```python
from build123d import *

# Parameters (mm, degrees)
SKETCH1_R           = 11
SKETCH1_R_2         = 1.5
SKETCH1_W           = 5
SKETCH1_H           = 6
BOSS_EXTRUDE1_DEPTH = 5


with BuildPart() as part:
    # Sketch1 → Boss-Extrude1 (new body)
    with BuildSketch(Plane(origin=(0, 0, 0), x_dir=(1, 0, 0), z_dir=(0, 1, 0))):
        with BuildLine():
            Line((48.7, 25.000004028), (38.700001305, 25.000004028))
            ThreePointArc((38.700001305, 25.000004028), (35.164467017, 23.535538857), (33.7, 20.000005334))
            Line((33.7, 20.000005334), (33.7, -25))
            ThreePointArc((33.7, -25), (35.164465799, -28.535533784), (38.699999411, -30))
            Line((38.699999411, -30), (54.2, -30))
            Line((54.2, -30), (54.2, -55))
            Line((54.2, -55), (41.099999997, -55))
            Line((41.099999997, -55), (41.099999997, -63))
            Line((41.099999997, -63), (-23.900000003, -63))
            Line((-23.900000003, -63), (-23.900000003, -55))
            Line((-23.900000003, -55), (-37.00036842, -55))
            ThreePointArc((-37.00036842, -55), (-42.656802211, -52.657122122), (-45.000000024, -47.000820858))
            Line((-45.000000024, -47.000820858), (-45.000000024, 15.001139744))
            ThreePointArc((-45.000000024, 15.001139744), (-36.213537283, 36.213537259), (-15.001139768, 45))
            Line((-15.001139768, 45), (48.7, 45))
            ThreePointArc((48.7, 45), (58.699997986, 35.000002014), (48.7, 25.000004028))
        make_face()
        Circle(SKETCH1_R, mode=Mode.SUBTRACT)
        with Locations((9.89288341, 9.906102051)):
            Circle(SKETCH1_R_2, mode=Mode.SUBTRACT)
        with Locations((9.89288341, -9.906102051)):
            Circle(SKETCH1_R_2, mode=Mode.SUBTRACT)
        with Locations((-9.89288341, -9.906102051)):
            Circle(SKETCH1_R_2, mode=Mode.SUBTRACT)
        with Locations((-9.89288341, 9.906102051)):
            Circle(SKETCH1_R_2, mode=Mode.SUBTRACT)
        with Locations((-9.400000003, -59)):
            Circle(SKETCH1_R_2, mode=Mode.SUBTRACT)
        with Locations((26.599999997, -59)):
            Circle(SKETCH1_R_2, mode=Mode.SUBTRACT)
        with Locations((48.7, 35.000002014)):
            Circle(SKETCH1_R_2, mode=Mode.SUBTRACT)
        with Locations((-30.000000024, -40)):
            Circle(SKETCH1_R_2, mode=Mode.SUBTRACT)
        with Locations((36.599999976, -40)):
            Circle(SKETCH1_R_2, mode=Mode.SUBTRACT)
        with Locations((-39.500000024, -31)):
            Rectangle(SKETCH1_W, SKETCH1_H, mode=Mode.SUBTRACT)
        with Locations((-39.500000024, -47)):
            Rectangle(SKETCH1_W, SKETCH1_H, mode=Mode.SUBTRACT)
        with Locations((48.7, -36)):
            Rectangle(SKETCH1_W, SKETCH1_H, mode=Mode.SUBTRACT)
        with Locations((48.7, -49)):
            Rectangle(SKETCH1_W, SKETCH1_H, mode=Mode.SUBTRACT)
    extrude(amount=BOSS_EXTRUDE1_DEPTH)


solid = part.part
```
Geometry check sheet. Reference: the model listing, model coordinates, mm. A direction names the side the tool comes from. Coordinates: 2 decimals unless noted, no trailing zeros. Write each loop counter-clockwise with the first axis right and the second up, starting at its lowest first coordinate (ties: lowest second). Pieces come first, ordered by that corner, then holes. Notation, with made-up numbers: M -4,17.25 L 13,17.25 A9 ccw 13,32.25 Z; hole C 86,65.5 d6. An arc over 180 degrees is marked long. Answer as a JSON object with one key per item and string values.
1. Section check D-D, the plane z = -17. Enter the section's corners in (x, y), plus the area to 3 significant figures.
Answers below:
{"outline": "M -44.93,0 L 33.7,0 L 33.7,5 L -44.93,5 Z", "area": "393 mm²"}
2. Section check B-B, the plane x = 36.6. Enter the section's corners in (y, z), plus the area to 3 significant figures.
Answers below:
{"outline": "M 0,-45 L 5,-45 L 5,-24.54 L 0,-24.54 Z; M 0,29.54 L 5,29.54 L 5,38.5 L 0,38.5 Z; M 0,41.5 L 5,41.5 L 5,63 L 0,63 Z", "area": "255 mm²"}
3. Tool access check on faces 4 (the flat face through (44, 2, -25)), 5 (the flat face through (-30, 2, 55)), 6 (the flat face through (48, 2, 55)), 7 (the flat face through (-40, 2, 50)). Record the directions out of +Z, -Z, +X, -X, +Y, -Y that give a thin tool (end or side, any length) a straight path to the whole face; none if there is none.
Answers below:
{"face 4": "+X, +Y, -Y", "face 5": "+Z, -X, +Y, -Y", "face 6": "+Z, +X, +Y, -Y", "face 7": "+Y, -Y"}
4. Go/stop test with flat-tipped pins: pin 1 Ø2.5 at (y, z) = (2, 2) entering from +X; pin 2 Ø2.5 at (x, y) = (49, 3) entering from +Z; pin 3 Ø1 at (y, z) = (4, -22) entering from +X; pin 4 Ø20 at (x, z) = (0, 0) entering from +Y. Record where each tip stops, or that it passes through.
Answers below:
{"pin 1": "stops at x = 33.7", "pin 2": "stops at z = 55", "pin 3": "stops at x = 34.37", "pin 4": "passes through"}
5. Scan lines: L1, parallel to X at y = 3.4, z = 59; L2, parallel to Z at x = 48.7, y = 3.9; L3, parallel to X at y = 0.3, z = 47.5. Record each from-to range of solid material in increasing order.
Answers below:
{"L1": "x = -23.9 to -10.9, -7.9 to 25.1, 28.1 to 41.1", "L2": "z = -45 to -36.5, -33.5 to -25, 30 to 33, 39 to 46, 52 to 55", "L3": "x = -44.98 to -42, -37 to 46.2, 51.2 to 54.2"}
6. Draft check along X on faces 1 (the flat face through (-40, 2, 34)), 2 (the cylindrical face through (-36.445, 2.465, -35.979)), 3 (the cylindrical face through (35.13, 2.46, 28.5)). Enter one of: released by +X, released by -X, zero draft, split by the parting line, or undercut.
Answers below:
{"face 1": "undercut", "face 2": "released by -X", "face 3": "released by +X"}
7. Section check C-C, the plane y = 3.6. Give the number of separate pieces and of enclosed holes in the cut face, plus the area to 3 significant figures.
Answers below:
{"separate pieces": "1", "enclosed holes": "14", "area": "8,600 mm²"}
8. Section check A-A, the plane z = 59. Enter the section's corners in (x, y), plus the area to 3 significant figures.
Answers below:
{"outline": "M -23.9,0 L -10.9,0 L -10.9,5 L -23.9,5 Z; M -7.9,0 L 25.1,0 L 25.1,5 L -7.9,5 Z; M 28.1,0 L 41.1,0 L 41.1,5 L 28.1,5 Z", "area": "295 mm²"}
